The model under review builds one solid part; all positions refer to its coordinate system, in mm. A direction names the side the tool comes from. Round coordinates to 2 decimals unless told otherwise and drop trailing zeros. Loops run counter-clockwise (first coordinate to the right, second up) from the corner with the lowest first, then second, coordinate; pieces in that order, holes last. Notation, with made-up numbers: M -30,22 L 6,22 A20 cw 6,43 Z; hole C 70,5.25 d3. An arc over 180 degrees is marked long. One line per question, with ' | ' between items.
from build123d import *

# Parameters (mm, degrees)
SKETCH1_R           = 15
SKETCH1_R_2         = 8
BOSS_EXTRUDE1_DEPTH = 80
SKETCH2_R           = 50
SKETCH2_R_2         = 12.5
BOSS_EXTRUDE2_DEPTH = 8
SKETCH3_R           = 2.5
CUT_EXTRUDE1_DEPTH  = 8
CIRPATTERN1_COUNT   = 3


with BuildPart() as part:
    # Sketch1 → Boss-Extrude1 (new body)
    with BuildSketch(Plane.XY.offset(10)):
        Circle(SKETCH1_R)
        Circle(SKETCH1_R_2, mode=Mode.SUBTRACT)
    extrude(amount=BOSS_EXTRUDE1_DEPTH)

    # Sketch2 → Boss-Extrude2 (add)
    with BuildSketch(Plane(origin=(0, 0, 10), x_dir=(-1, 0, 0), z_dir=(0, 0, -1))):
        Circle(SKETCH2_R)
        Circle(SKETCH2_R_2, mode=Mode.SUBTRACT)
    extrude(amount=-BOSS_EXTRUDE2_DEPTH)

    # Sketch3 → Cut-Extrude1 (cut)
    with BuildSketch(Plane.XY.offset(18)):
        with Locations((0, 40)):
            Circle(SKETCH3_R)
    cut_extrude1 = extrude(amount=-CUT_EXTRUDE1_DEPTH, mode=Mode.SUBTRACT)

    # CirPattern1: Cut-Extrude1 ×3 about axis
    cirpattern1_axis = Axis((0, 0, 0), (0, 0, 1))
    for i in range(1, CIRPATTERN1_COUNT):
        add(cut_extrude1.rotate(cirpattern1_axis, i * 360 / CIRPATTERN1_COUNT), mode=Mode.SUBTRACT)


solid = part.part
1) For line 1 (Z direction, x = 6, y = 33); line 2 (Y direction, x = 0, z = 64); line 3 (X direction, y = -2, z = 77), list the stretches that pass through material, from the lowest coordinate up.
Output values:
line 1: z = 10 to 18 | line 2: y = -15 to -8, 8 to 15 | line 3: x = -14.87 to -7.75, 7.75 to 14.87
2) Add section C-C on y = -20. State the section outline as (x, z) points.
Output values:
outline: M -45.83,10 L -37.14,10 L -37.14,18 L -45.83,18 Z; M -32.14,10 L 32.14,10 L 32.14,18 L -32.14,18 Z; M 37.14,10 L 45.83,10 L 45.83,18 L 37.14,18 Z
3) Add section A-A on y = 0. State the section outline as (x, z) points, then the cut area to 3 significant figures.
Output values:
outline: M -50,10 L -8,10 L -8,90 L -15,90 L -15,18 L -50,18 Z; M 8,10 L 50,10 L 50,18 L 15,18 L 15,90 L 8,90 Z | area: 1,680 mm²
4) Machinability: for faces 5 (the flat face through (-10, 12, 18)), 6 (the cylindrical face through (-1.73, -7.81, 49.44)), which of the approach directions +Z, -Z, +X, -X, +Y, -Y give a long, thin tool a straight path to every point of the face, cutting with its end or side? Answer none if there is none.
Output values:
face 5: +Z | face 6: +Z, -Z
5) Add section B-B on x = 0. State the section outline as (y, z) points.
Output values:
outline: M -50,10 L -8,10 L -8,90 L -15,90 L -15,18 L -50,18 Z; M 8,10 L 37.5,10 L 37.5,18 L 15,18 L 15,90 L 8,90 Z; M 42.5,10 L 50,10 L 50,18 L 42.5,18 Z
6) Insertion check: P1, Ø6, axis at x = -34.64, y = -20, coming from the +Z side. The pin has a flat end and moves straight along its axis. Give the tip position at first contact, or say it passes through.
Output values:
P1: stops at z = 18
7) Add section D-D on z = 41. State the section outline as (x, y) points, then the cut area to 3 significant figures.
Output values:
outline: C 0,0 d30; hole C 0,0 d16 | area: 506 mm²
8) Mouldability with a two-part tool opening along Y and no side actions: class faces 1 (the cylindrical face through (-34.97, -17.52, 14.06)), 2 (the cylindrical face through (32.8, -18.31, 14.06)), 3 (the cylindrical face through (-14.985, 0.66, 53.496)), 4 (the flat face through (6, -6, 90)) as +Y half, -Y half, draft (parallel to the pull), parting line (faces both ways), or undercut.
Output values:
face 1: undercut | face 2: undercut | face 3: parting line | face 4: draft
